Can you work these out from the model? Positions are in its coordinate system, mm. A direction names the side the tool comes from. Give positions to 0.01 mm unless a question says otherwise; leave off trailing zeros. Loops run counter-clockwise (first coordinate to the right, second up) from the corner with the lowest first, then second, coordinate; pieces in that order, holes last. Notation, with made-up numbers: (69.5, 82) -> (85.5, 82) arc R20 ccw to (85.5, 96) -> close; hole circle Ø5 at (-36, 19.25). An arc over 180 degrees is marked (long way). Use CSV: the item, a comma, the result in double quotes.
from build123d import *

# Parameters (mm, degrees)
BANDAID_START                  = 0.053848
SKETCH3_R                      = 30.84068
SKETCH3_R_2                    = 15.875
BANDAID_SOLUTION_THICKER_DEPTH = 0.053848
SKETCH4_R                      = 22.86
SKETCH4_R_2                    = 15.875
LIP_FOR_BEARING_DEPTH          = 1.016


with BuildPart() as part:
    # Sketch1 → Revolve1 (revolve)
    with BuildSketch(Plane(origin=(0, 0, 0), x_dir=(0, 0, -1), z_dir=(1, 0, 0))):
        Polygon((-15.875, 2.694084), (-15.875, -5.020818), (-30.84068, -5.020818), (-30.84068, -1.062068), (-29.43479, -1.062068), (-29.43479, 1.477932), (-30.84068, 1.477932), (-30.84068, 2.694084), align=None)
    revolve(axis=Axis((0, 0, 0), (0, -1, 0)))

    # Sketch3 → BandAid Solution thicker (add)
    with BuildSketch(Plane(origin=(0, 2.694084, 0), x_dir=(1, 0, 0), z_dir=(0, 1, 0)).offset(BANDAID_START)):
        with Locations(Location((0, 0, 0), (0, 0, 270))):
            Circle(SKETCH3_R)
        with Locations(Location((0, 0, 0), (0, 0, 270))):
            Circle(SKETCH3_R_2, mode=Mode.SUBTRACT)
    extrude(amount=-BANDAID_SOLUTION_THICKER_DEPTH)

    # Sketch4 → Lip for Bearing (add)
    with BuildSketch(Plane(origin=(0, 2.747932, 0), x_dir=(1, 0, 0), z_dir=(0, 1, 0))):
        with Locations(Location((0, 0, 0), (0, 0, 90))):
            Circle(SKETCH4_R)
        with Locations(Location((0, 0, 0), (0, 0, 270))):
            Circle(SKETCH4_R_2, mode=Mode.SUBTRACT)
    extrude(amount=LIP_FOR_BEARING_DEPTH)


solid = part.part
(1) Will these pins go through, and if not, where does the flat tip stop? pin 1 Ø19 at (x, z) = (0, 0) entering from +Y; pin 2 Ø1 at (x, y) = (21, -2.5) entering from -Z; pin 3 Ø10 at (x, z) = (20.5, 20.5) entering from +Y.
Answer sheet:
pin 1,"passes through"
pin 2,"stops at z = -23.04"
pin 3,"stops at y = 2.75"
(2) We'd pull the mould along Y, two halves only. Please class faces 1 (the face through (-11, 2.748, -21)), 2 (the face through (25, 1.478, -16)), 3 (the face through (-22.665, 3.249, 2.976)): released by +Y, released by -Y, zero draft, split by the parting line, or undercut.
Answer sheet:
face 1,"released by +Y"
face 2,"undercut"
face 3,"zero draft"
(3) Which directions (+Z, -Z, +X, -X, +Y, -Y) give clear straight access to the entire face, cutting with the end or side of a thin tool? Please do faces 4 (the face through (17.91, 0.23, -23.36)), 5 (the face through (-9.264, -3.014, 29.417)).
Answer sheet:
face 4,"none"
face 5,"+Y, -Y"
(4) If I drill on L1, parallel to Z at x = 0, y = -3.25 (3 decimals); L2, parallel to X at y = 3.2, z = 0 (3 decimals), over which ranges is the centre line in solid material (lowest first)? Write a range as from..to.
Answer sheet:
L1,"z = -30.841..-15.875, 15.875..30.841"
L2,"x = -22.86..-15.875, 15.875..22.86"
(5) If we section it at D-D, the plane z = 20: Write out the boundary of the cut face in (x, y), then the cut area to 3 significant figures.
Answer sheet:
outline,"(-23.48, -5.02) -> (23.48, -5.02) -> (23.48, -1.06) -> (21.6, -1.06) -> (21.6, 1.48) -> (23.48, 1.48) -> (23.48, 2.75) -> (11.07, 2.75) -> (11.07, 3.76) -> (-11.07, 3.76) -> (-11.07, 2.75) -> (-23.48, 2.75) -> (-23.48, 1.48) -> (-21.6, 1.48) -> (-21.6, -1.06) -> (-23.48, -1.06) -> close"
area,"378 mm2"
(6) If we section it at A-A, the plane x = 0: Write out the boundary of the cut face in (y, z) (3 decimals), then the cut area to 3 significant figures.
Answer sheet:
outline,"(-5.021, -30.841) -> (-1.062, -30.841) -> (-1.062, -29.435) -> (1.478, -29.435) -> (1.478, -30.841) -> (2.748, -30.841) -> (2.748, -22.86) -> (3.764, -22.86) -> (3.764, -15.875) -> (-5.021, -15.875) -> close; (-5.021, 15.875) -> (3.764, 15.875) -> (3.764, 22.86) -> (2.748, 22.86) -> (2.748, 30.841) -> (1.478, 30.841) -> (1.478, 29.435) -> (-1.062, 29.435) -> (-1.062, 30.841) -> (-5.021, 30.841) -> close"
area,"240 mm2"
(7) If we section it at B-B, the plane z = 0: Write out the boundary of the cut face in (x, y) (3 decimals).
Answer sheet:
outline,"(-30.841, -5.021) -> (-15.875, -5.021) -> (-15.875, 3.764) -> (-22.86, 3.764) -> (-22.86, 2.748) -> (-30.841, 2.748) -> (-30.841, 1.478) -> (-29.435, 1.478) -> (-29.435, -1.062) -> (-30.841, -1.062) -> close; (15.875, -5.021) -> (30.841, -5.021) -> (30.841, -1.062) -> (29.435, -1.062) -> (29.435, 1.478) -> (30.841, 1.478) -> (30.841, 2.748) -> (22.86, 2.748) -> (22.86, 3.764) -> (15.875, 3.764) -> close"
(8) If we section it at C-C, the plane y = -3.5: Write out the boundary of the cut face in (x, z) (3 decimals), then the cut area to 3 significant figures.
Answer sheet:
outline,"circle Ø61.681 at (0, 0); hole circle Ø31.75 at (0, 0)"
area,"2,200 mm2"
